Here's how the part is built. I have some questions about the finished solid (model axes, mm). Face numbers are marked on the shaded views. Give positions to 0.01 mm unless a question says otherwise; leave off trailing zeros. Loops run counter-clockwise (first coordinate to the right, second up) from the corner with the lowest first, then second, coordinate; pieces in that order, holes last. Notation, with made-up numbers: (45, 57) - (85, 57) arc R34 cw to (85, 89) - close; hole circle Ø9 at (81.25, 32). An arc over 180 degrees is marked (long way). Use a Markdown table: item, result.
from build123d import *

# Parameters (mm, degrees)
EXTRUDE_1_DEPTH    = 11
HOLE_WIZARD_M3_1_D = 2.5


with BuildPart() as part:
    # 草图1 → 凸台-拉伸1 (new body, symmetric)
    with BuildSketch(Plane.XY):
        Polygon((1.356773133, 2.35), (-1.356773133, 2.35), (-2.713546265, 0), (-1.356773133, -2.35), (1.356773133, -2.35), (2.713546265, 0), align=None)
    extrude(amount=EXTRUDE_1_DEPTH, both=True)

    # M3 螺纹孔1 (through all)
    with Locations(Plane.XY.offset(11)):
        with Locations((0, 0)):
            Hole(HOLE_WIZARD_M3_1_D / 2)


solid = part.part
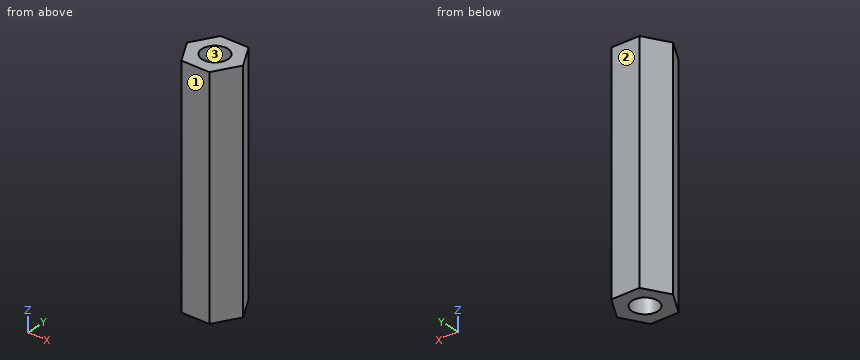
(1) We'd pull the mould along Y, two halves only. Please class the marked faces 1, 2 and 3: pulls with the +Y half, pulls with the -Y half, needs draft (parallel to the pull), parting line crosses it, or undercut.
A:
| item | result |
|---|---|
| face 1 | pulls with the -Y half |
| face 2 | pulls with the +Y half |
| face 3 | undercut |
(2) Suppose I cut it at C-C on z = 9.75. Write out the boundary of the cut face in (x, y).
A:
| item | result |
|---|---|
| outline | (-2.71, 0) - (-1.36, -2.35) - (1.36, -2.35) - (2.71, 0) - (1.36, 2.35) - (-1.36, 2.35) - close; hole circle Ø2.5 at (0, 0) |
(3) Suppose I cut it at D-D on x = 2.15. Write out the boundary of the cut face in (y, z).
A:
| item | result |
|---|---|
| outline | (-0.98, -11) - (0.98, -11) - (0.98, 11) - (-0.98, 11) - close |
(4) Suppose I cut it at B-B on y = 0.3. Write out the boundary of the cut face in (x, z), plus the area to 3 significant figures.
A:
| item | result |
|---|---|
| outline | (-2.54, -11) - (-1.21, -11) - (-1.21, 11) - (-2.54, 11) - close; (1.21, -11) - (2.54, -11) - (2.54, 11) - (1.21, 11) - close |
| area | 58.4 mm2 |
(5) Suppose I cut it at A-A on x = 0. Write out the boundary of the cut face in (y, z).
A:
| item | result |
|---|---|
| outline | (-2.35, -11) - (-1.25, -11) - (-1.25, 11) - (-2.35, 11) - close; (1.25, -11) - (2.35, -11) - (2.35, 11) - (1.25, 11) - close |
(6) If I drill on line 1 (Y direction, x = 0, z = 2.75); line 2 (Y direction, x = -1, z = 10); line 3 (X direction, y = 1, z = -9), over which ranges is the centre line in solid material (lowest first)?
A:
| item | result |
|---|---|
| line 1 | -2.35 to -1.25, 1.25 to 2.35 |
| line 2 | -2.35 to -0.75, 0.75 to 2.35 |
| line 3 | -2.14 to -0.75, 0.75 to 2.14 |
(7) Will this pin go through, and if not, where does the flat tip stop? pin 1 (1.5 mm diameter, centred on x = 2, z = 6.5, fed in from +Y).
A:
| item | result |
|---|---|
| pin 1 | y = 2.35 |
